Print and shaded views of the part. All mm, measured from the part's lowest x, y and z. Give positions to 0.01 mm unless a question says otherwise; leave off trailing zeros. Order: outer loops, then holes, each group sorted by start corner. A loop starts at its lowest first (then second) coordinate and runs counter-clockwise, first axis right, second up. Notation, with made-up numbers: (-19.75, 24) -> (16.25, 24) arc R19 ccw to (16.25, 30) -> close; hole circle Ø11 at (35.25, 44.25). An arc over 180 degrees is marked (long way). One line per question, with ' | ' between items. Start each with the question number.
(1) Cut at C-C (z = 0.25). Give the cut face in (x, y), then the cut area to 3 significant figures.
(2) Drill centre lines: L1, parallel to Y at x = 4.5, z = 0.35; L2, parallel to Y at x = 30.5, z = 0.4; L3, parallel to X at y = 42.5, z = 0.35. Where is each one in solid material? Low to high. Write a range as from..to.
(3) Cut at D-D (y = 4.5). Give the cut face in (x, z).
(4) Cut at A-A (x = 30.5). Give the cut face in (y, z), then the cut area to 3 significant figures.
(5) Cut at B-B (y = 29.5). Give the cut face in (x, z), then the cut area to 3 significant figures.
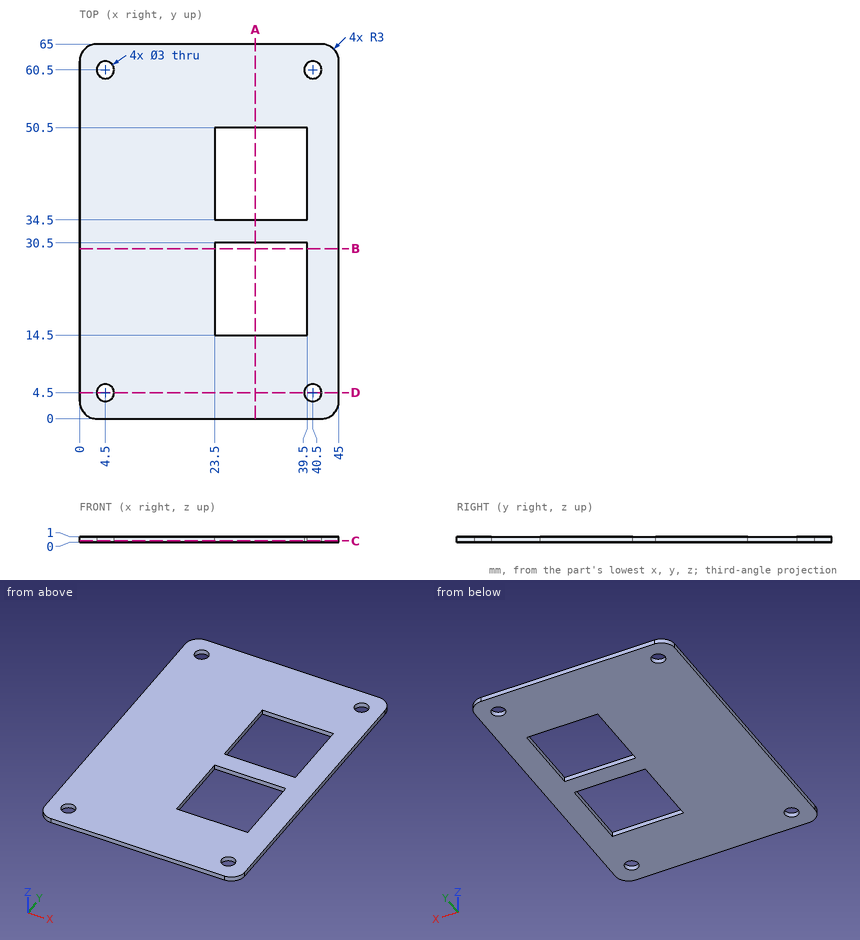
Result set:
1) outline: (0, 3) arc R3 ccw to (3, 0) -> (42, 0) arc R3 ccw to (45, 3) -> (45, 62) arc R3 ccw to (42, 65) -> (3, 65) arc R3 ccw to (0, 62) -> close; hole circle Ø3 at (4.5, 4.5); hole circle Ø3 at (4.5, 60.5); hole (23.5, 14.5) -> (39.5, 14.5) -> (39.5, 30.5) -> (23.5, 30.5) -> close; hole (23.5, 34.5) -> (39.5, 34.5) -> (39.5, 50.5) -> (23.5, 50.5) -> close; hole circle Ø3 at (40.5, 4.5); hole circle Ø3 at (40.5, 60.5) | area: 2,380 mm2
2) L1: y = 0..3, 6..59, 62..65 | L2: y = 0..14.5, 30.5..34.5, 50.5..65 | L3: x = 0..23.5, 39.5..45
3) outline: (0, 0) -> (3, 0) -> (3, 1) -> (0, 1) -> close; (6, 0) -> (39, 0) -> (39, 1) -> (6, 1) -> close; (42, 0) -> (45, 0) -> (45, 1) -> (42, 1) -> close
4) outline: (0, 0) -> (14.5, 0) -> (14.5, 1) -> (0, 1) -> close; (30.5, 0) -> (34.5, 0) -> (34.5, 1) -> (30.5, 1) -> close; (50.5, 0) -> (65, 0) -> (65, 1) -> (50.5, 1) -> close | area: 33.0 mm2
5) outline: (0, 0) -> (23.5, 0) -> (23.5, 1) -> (0, 1) -> close; (39.5, 0) -> (45, 0) -> (45, 1) -> (39.5, 1) -> close | area: 29.0 mm2
